Geometry check sheet. Reference: drawing and pictorial views, mm from the part's lowest x, y, z. A direction names the side the tool comes from. Give positions to 0.01 mm unless a question says otherwise; leave off trailing zeros. Loops run counter-clockwise (first coordinate to the right, second up) from the corner with the lowest first, then second, coordinate; pieces in that order, holes last. Notation, with made-up numbers: (28.25, 60.25) -> (67.25, 60.25) arc R27 cw to (67.25, 99.25) -> close; hole circle Ø1 at (-39, -1). An arc over 180 degrees is marked (long way). Answer in a Markdown table with one row per item. Add a question column.
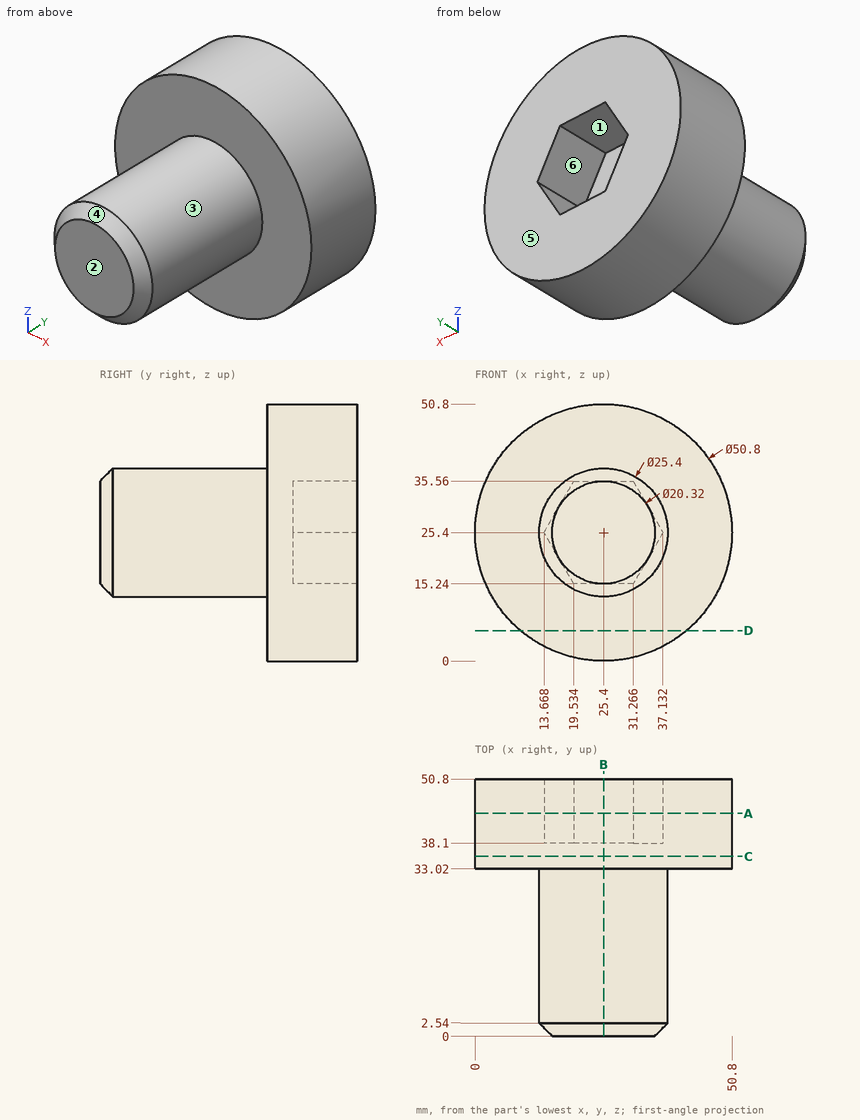
1. Access from +Z, -Z, +X, -X, +Y, -Y to the whole of each face (thin tool, end or side, straight path). Record for the marked faces 1, 2 and 3.
2. Material ranges on L1, parallel to Y at x = 5.5, z = 38; L2, parallel to Y at x = 31, z = 26; L3, parallel to X at y = 43.5, z = 31.5, recorded low to high. Write a range as from..to.
3. Sectioned sample at B-B (x = 25.4). Enter the section's corners in (y, z), plus the area to 3 significant figures.
4. Gauge pin test, flat ends, axial feed: pin 1 Ø3 at (x, y) = (42.5, 34) entering from -Z (1 decimal); pin 2 Ø6 at (x, y) = (28, 41.5) entering from +Z; pin 3 Ø2 at (x, y) = (26, 8) entering from +Z. Record the tip position at first contact, or that the pin passes through.
5. Sectioned sample at D-D (z = 6). Enter the section's corners in (x, y) (1 decimal).
6. Sectioned sample at A-A (y = 44). Enter the section's corners in (x, z), plus the area to 3 significant figures.
7. Release check for a two-part mould opening along Z. For the marked faces 4, 5 and 6 record: released by +Z, released by -Z, zero draft, split by the parting line, or undercut.
8. Sectioned sample at C-C (y = 35.5). Enter the section's corners in (x, z).
Response:
| question | item | result |
|---|---|---|
| 1 | face 1 | +Y |
| 1 | face 2 | +Z, -Z, +X, -X, -Y |
| 1 | face 3 | -Y |
| 2 | L1 | y = 33.02..50.8 |
| 2 | L2 | y = 0..38.1 |
| 2 | L3 | x = 0.74..17.19, 33.61..50.06 |
| 3 | outline | (0, 15.24) -> (2.54, 12.7) -> (33.02, 12.7) -> (33.02, 0) -> (50.8, 0) -> (50.8, 15.24) -> (38.1, 15.24) -> (38.1, 35.56) -> (50.8, 35.56) -> (50.8, 50.8) -> (33.02, 50.8) -> (33.02, 38.1) -> (2.54, 38.1) -> (0, 35.56) -> close |
| 3 | area | 1,480 mm2 |
| 4 | pin 1 | stops at z = 5.4 |
| 4 | pin 2 | stops at z = 50.8 |
| 4 | pin 3 | stops at z = 38.1 |
| 5 | outline | (9, 33) -> (41.8, 33) -> (41.8, 50.8) -> (9, 50.8) -> close |
| 6 | outline | circle Ø50.8 at (25.4, 25.4); hole (13.67, 25.4) -> (19.53, 15.24) -> (31.27, 15.24) -> (37.13, 25.4) -> (31.27, 35.56) -> (19.53, 35.56) -> close |
| 6 | area | 1,670 mm2 |
| 7 | face 4 | split by the parting line |
| 7 | face 5 | zero draft |
| 7 | face 6 | undercut |
| 8 | outline | circle Ø50.8 at (25.4, 25.4) |
